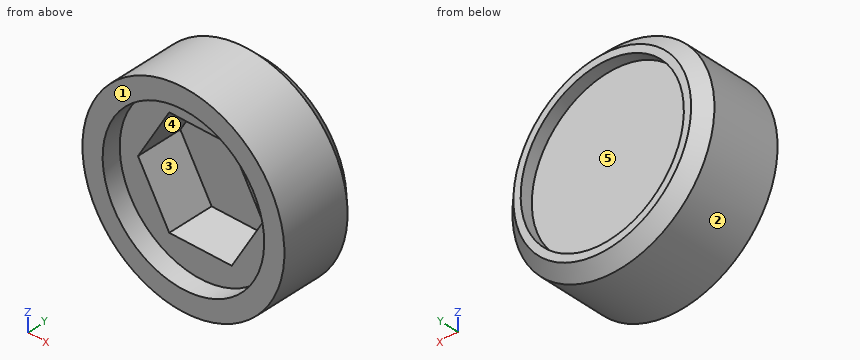
from build123d import *

# Parameters (mm, degrees)
SKETCH1_R           = 12.5
BOSS_EXTRUDE1_DEPTH = 10
CUT_EXTRUDE1_DEPTH  = 8
CHAMFER1_SIZE       = 1.5
SKETCH5_R           = 10
CUT_EXTRUDE2_DEPTH  = 6
SKETCH6_R           = 10.1
CUT_EXTRUDE3_DEPTH  = 1.5


with BuildPart() as part:
    # Sketch1 → Boss-Extrude1 (new body)
    with BuildSketch(Plane(origin=(0, 0, 0), x_dir=(1, 0, 0), z_dir=(0, 1, 0))):
        with Locations(Location((0, 0, 0), (0, 0, 270))):
            Circle(SKETCH1_R)
    extrude(amount=BOSS_EXTRUDE1_DEPTH)

    # Sketch2 → Cut-Extrude1 (cut)
    with BuildSketch(Plane.XZ):
        Polygon((7.736493607, 0), (3.868246804, 6.7), (-3.868246804, 6.7), (-7.736493607, 0), (-3.868246804, -6.7), (3.868246804, -6.7), align=None)
    extrude(amount=-CUT_EXTRUDE1_DEPTH, mode=Mode.SUBTRACT)

    # Chamfer1
    chamfer1_edges = [part.edges().sort_by_distance(p)[0] for p in [
        (0, 10, -12.5),
    ]]
    chamfer(chamfer1_edges, length=CHAMFER1_SIZE)

    # Sketch5 → Cut-Extrude2 (cut)
    with BuildSketch(Plane(origin=(0, 2.3, 0), x_dir=(-1, 0, 0), z_dir=(0, -1, 0))):
        with Locations(Location((0, 0, 0), (0, 0, 270))):
            Circle(SKETCH5_R)
    extrude(amount=CUT_EXTRUDE2_DEPTH, mode=Mode.SUBTRACT)

    # Sketch6 → Cut-Extrude3 (cut)
    with BuildSketch(Plane(origin=(0, 10, 0), x_dir=(1, 0, 0), z_dir=(0, 1, 0))):
        with Locations(Location((0, 0, 0), (0, 0, 270))):
            Circle(SKETCH6_R)
    extrude(amount=-CUT_EXTRUDE3_DEPTH, mode=Mode.SUBTRACT)


solid = part.part
Read the model definition and answer for the solid it produces. Units are mm, in the model's axes. Face numbers are marked on the shaded views. A direction names the side the tool comes from. Round coordinates to 2 decimals unless told otherwise and drop trailing zeros. Write each loop counter-clockwise with the first axis right and the second up, starting at its lowest first coordinate (ties: lowest second). Pieces come first, ordered by that corner, then holes.
1. The part is cut by section C-C, the plane y = 1.75. Determine the outline of the cut face in (x, z), then the cut area to 3 significant figures.
2. Straight lines are drawn through the part: L1, parallel to X at y = 1.2, z = 0; L2, parallel to X at y = 4.5, z = 6; L3, parallel to Y at x = 4.75, z = 7.5. For each, find the intervals that lie inside material, in ascending order.
3. Given pin 1 Ø1.7 at (x, y) = (1, 4.5) entering from -Z; pin 2 Ø1 at (x, y) = (-3, 1.5) entering from -Z; pin 3 Ø10 at (x, z) = (2.5, 1.5) entering from +Y, each flat-ended and moving along its own axis, determine where each tip first touches the part or whether it passes through.
4. The part is cut by section A-A, the plane y = 4.5. Determine the outline of the cut face in (x, z).
5. Determine the mould class of the marked faces 1, 2 and 3 for opening direction Z: pulls with the +Z half, pulls with the -Z half, needs draft (parallel to the pull), parting line crosses it, or undercut.
6. The part is cut by section B-B, the plane x = 0. Determine the outline of the cut face in (y, z).
7. Which of the six approach directions +Z, -Z, +X, -X, +Y, -Y give full straight-line access (tool end or side, diameter ignored) to the marked faces 4 and 5?
Values:
1. outline: circle Ø25 at (0, 0); hole circle Ø20 at (0, 0)
1. area: 177 mm2
2. L1: x = -12.5 to -10, 10 to 12.5
2. L2: x = -10.97 to -4.27, 4.27 to 10.97
2. L3: y = 2.3 to 8.5
3. pin 1: stops at z = -12.5
3. pin 2: stops at z = -12.25
3. pin 3: stops at y = 8.5
4. outline: circle Ø25 at (0, 0); hole (-7.74, 0) - (-3.87, -6.7) - (3.87, -6.7) - (7.74, 0) - (3.87, 6.7) - (-3.87, 6.7) - close
5. face 1: needs draft
5. face 2: parting line crosses it
5. face 3: undercut
6. outline: (0, -12.5) - (8.5, -12.5) - (10, -11) - (10, -10.1) - (8.5, -10.1) - (8.5, 10.1) - (10, 10.1) - (10, 11) - (8.5, 12.5) - (0, 12.5) - (0, 10) - (2.3, 10) - (2.3, 6.7) - (8, 6.7) - (8, -6.7) - (2.3, -6.7) - (2.3, -10) - (0, -10) - close
7. face 4: -Y
7. face 5: +Y
